Geometry: see drawing. Coordinates: mm, zero at the bounding-box minimum. Give positions to 0.01 mm unless a question says otherwise; leave off trailing zeros. Order: outer loops, then holes, each group sorted by start corner. A loop starts at its lowest first (then second) coordinate and runs counter-clockwise, first axis right, second up. Notation, with made-up numbers: M 36.5,-7 L 69.5,-7 A13 ccw 69.5,0 Z; hole C 19.5,2 d9. An arc over 180 degrees is marked long. Answer as a JSON object with one key per item and string values. Group by question number.
1. Section query A-A (z = 35). Output: boundary loops of the cut face in (x, y), plus the area to 3 significant figures.
2. Pin query (flat end, axial travel): P1, Ø8, axis at x = 36, z = 54.5, coming from the -Y side; P2, Ø1.7, axis at y = 10.5, z = 28.5, coming from the -X side; P3, Ø10, axis at y = 370.5, z = 45.5, coming from the +X side. Return the tip coordinate at first contact, or that it passes through.
3. Material intervals for L1, parallel to Y at x = 38, z = 60; L2, parallel to Z at x = 34.5, y = 261; L3, parallel to X at y = 321, z = 33, sorted ascending. Write a range as [from, to].
4. Section query B-B (y = 295). Output: boundary loops of the cut face in (x, z), plus the area to 3 significant figures.
5. Section query D-D (z = 56). Output: boundary loops of the cut face in (x, y), plus the area to 3 significant figures.
6. Section query C-C (x = 21.5). Output: boundary loops of the cut face in (y, z).
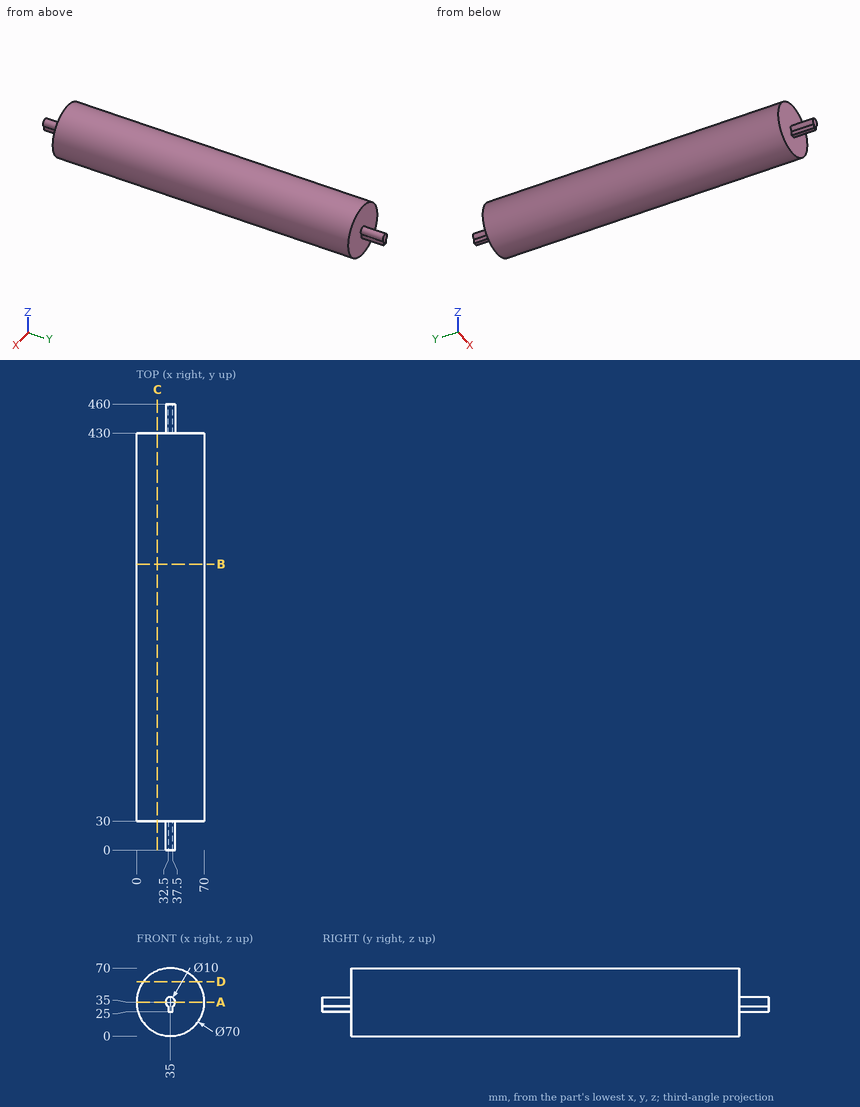
Answer sheet:
{
 "1": {"outline": "M 0,30 L 30,30 L 30,0 L 40,0 L 40,30 L 70,30 L 70,430 L 40,430 L 40,460 L 30,460 L 30,430 L 0,430 Z", "area": "28,600 mm^2"},
 "2": {"P1": "y = 30", "P2": "x = 32.5", "P3": "x = 69.57"},
 "3": {"L1": "[30, 430]", "L2": "[0, 70]", "L3": "[0.06, 69.94]"},
 "4": {"outline": "C 35,35 d70", "area": "3,850 mm^2"},
 "5": {"outline": "M 7,30 L 63,30 L 63,430 L 7,430 Z", "area": "22,400 mm^2"},
 "6": {"outline": "M 30,2.71 L 430,2.71 L 430,67.29 L 30,67.29 Z"}
}
